Here's how the part is built. I have some questions about the finished solid (model axes, mm). Face numbers are marked on the shaded views. A direction names the side the tool comes from. Round coordinates to 2 decimals unless told otherwise and drop trailing zeros. Loops run counter-clockwise (first coordinate to the right, second up) from the corner with the lowest first, then second, coordinate; pieces in that order, holes last. Notation, with made-up numbers: (40, 6) -> (88, 6) arc R15 cw to (88, 17) -> close; hole circle Ø6 at (50, 4). An arc over 180 degrees is marked (long way). Use one line per item in the form item = value. Start each with the question number.
Item 1: If we section it at D-D (z = 39.37): Write out the boundary of the cut face in (x, y), then the cut area to 3 significant figures.
Item 2: I'm going to push flat-ended pins straight in: pin 1 Ø3 at (x, y) = (10.5, 10.5) entering from -Z; pin 2 Ø3 at (y, z) = (-0.5, 37.5) entering from -X; pin 3 Ø1.6 at (y, z) = (0, 46.99) entering from +X. Where does each tip first touch, or does it pass through?
Item 3: If we section it at A-A (y = 6.5): Write out the boundary of the cut face in (x, z).
Item 4: For the marked faces 4 and 5, which set-ups out of +Z, -Z, +X, -X, +Y, -Y let a thin tool reach every point of the face, with its end or its side?
Item 5: If I drill on L1, parallel to Y at x = -11.5, z = 34.5; L2, parallel to Y at x = -14.75, z = 39.37, over which ranges is the centre line in solid material (lowest first)? Write a range as [from, to].
Item 6: If we section it at B-B (y = 0): Write out the boundary of the cut face in (x, z), then the cut area to 3 significant figures.
Item 7: Thinking about a two-plate mould opening in Y: for the marked faces 1, 2 and 3, which applies, released by +Y, released by -Y, zero draft, split by the parting line, or undercut?
```python
from build123d import *

# Parameters (mm, degrees)
BOSS_EXTRUDE1_DEPTH       = 76.2
BOSS_EXTRUDE1_DEPTH_BACK  = 76.2
SKETCH3_W                 = 38.1
SKETCH3_H                 = 38.1
SKETCH3_W_2               = 25.4
SKETCH3_H_2               = 25.4
SKETCH4_W                 = 38.1
SKETCH4_H                 = 38.1
SKETCH4_W_2               = 25.4
SKETCH4_H_2               = 25.4
CUT_EXTRUDE1_DEPTH        = 95.25
CUT_EXTRUDE4_REACH        = 89.298
SKETCH7_R                 = 3.81
F_6_32_TAPPED_HOLE1_D     = 2.7051
F_6_32_TAPPED_HOLE1_DEPTH = 6.35


with BuildPart() as part:
    # Sketch3 → Boss-Extrude1 (new, two sides: drawn at the far end of the back side and taken through both)
    with BuildSketch(Plane.XY.offset(-BOSS_EXTRUDE1_DEPTH_BACK)):
        Rectangle(SKETCH3_W, SKETCH3_H)
        Rectangle(SKETCH3_W_2, SKETCH3_H_2, mode=Mode.SUBTRACT)
    extrude(amount=BOSS_EXTRUDE1_DEPTH + BOSS_EXTRUDE1_DEPTH_BACK)

    # Sketch4 → Cut-Extrude1 (cut)
    with BuildSketch(Plane(origin=(0, 0, -76.2), x_dir=(-1, 0, 0), z_dir=(0, 0, -1))):
        Rectangle(SKETCH4_W, SKETCH4_H)
        Rectangle(SKETCH4_W_2, SKETCH4_H_2, mode=Mode.SUBTRACT)
    extrude(amount=-CUT_EXTRUDE1_DEPTH, mode=Mode.SUBTRACT)

    # Sketch7 → Cut-Extrude4 (cut, up to next)
    with BuildSketch(Plane(origin=(-19.05, 0, 0), x_dir=(0, -1, 0), z_dir=(-1, 0, 0)), mode=Mode.PRIVATE) as cut_extrude4_sk1:
        with Locations(Location((0, 39.37, 0), (0, 0, 90))):
            Circle(SKETCH7_R)
    cut_extrude4_tool1 = extrude(cut_extrude4_sk1.sketch, amount=-CUT_EXTRUDE4_REACH, mode=Mode.PRIVATE) & part.part
    add(cut_extrude4_tool1.solids().sort_by_distance((-19.05, 0, 39.37))[0], mode=Mode.SUBTRACT)

    # #6-32 Tapped Hole1
    with Locations(Plane(origin=(19.05, 0, 0), x_dir=(0, 0, -1), z_dir=(1, 0, 0))):
        with Locations((-29.21, 0), (-46.99, 0)):
            Hole(F_6_32_TAPPED_HOLE1_D / 2, depth=F_6_32_TAPPED_HOLE1_DEPTH)


solid = part.part
```
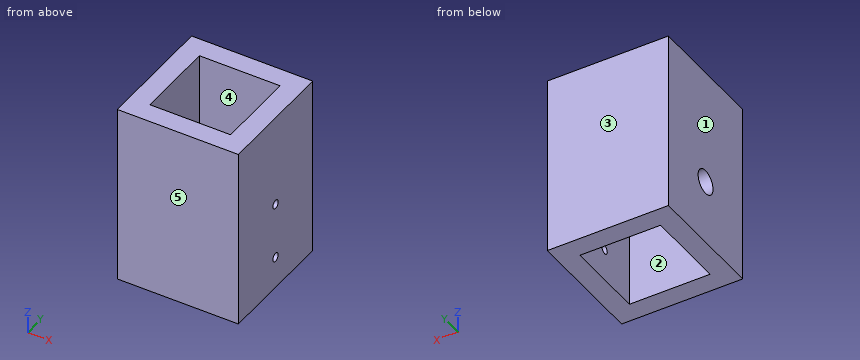
Values found:
q1.outline = (-19.05, -19.05) -> (19.05, -19.05) -> (19.05, 19.05) -> (-19.05, 19.05) -> (-19.05, 3.81) -> (-12.7, 3.81) -> (-12.7, 12.7) -> (12.7, 12.7) -> (12.7, -12.7) -> (-12.7, -12.7) -> (-12.7, -3.81) -> (-19.05, -3.81) -> close
q1.area = 758 mm2
q2.pin_1 = through
q2.pin_2 = 12.7
q2.pin_3 = -12.7
q3.outline = (-19.05, 19.05) -> (-12.7, 19.05) -> (-12.7, 76.2) -> (-19.05, 76.2) -> close; (12.7, 19.05) -> (19.05, 19.05) -> (19.05, 76.2) -> (12.7, 76.2) -> close
q4.face_4 = +Z, -Z
q4.face_5 = +Z, -Z, +X, -X, -Y
q5.L1 = [-19.05, -12.7], [12.7, 19.05]
q5.L2 = [-19.05, -3.81], [3.81, 19.05]
q6.outline = (-19.05, 19.05) -> (-12.7, 19.05) -> (-12.7, 35.56) -> (-19.05, 35.56) -> close; (-19.05, 43.18) -> (-12.7, 43.18) -> (-12.7, 76.2) -> (-19.05, 76.2) -> close; (12.7, 19.05) -> (19.05, 19.05) -> (19.05, 27.86) -> (12.7, 27.86) -> close; (12.7, 30.56) -> (19.05, 30.56) -> (19.05, 45.64) -> (12.7, 45.64) -> close; (12.7, 48.34) -> (19.05, 48.34) -> (19.05, 76.2) -> (12.7, 76.2) -> close
q6.area = 643 mm2
q7.face_1 = zero draft
q7.face_2 = undercut
q7.face_3 = released by +Y
